from build123d import *

# Parameters (mm, degrees)
SKETCH1_R             = 1.55
BOSS_EXTRUDE1_DEPTH   = 1.6
SKETCH1_3_R           = 1.55
BOSS_EXTRUDE2_DEPTH   = 4
BOSS_EXTRUDE2_2_DEPTH = 4
BOSS_EXTRUDE2_3_DEPTH = 4
BOSS_EXTRUDE2_4_DEPTH = 4
SKETCH1_4_R           = 1.55
BOSS_EXTRUDE3_DEPTH   = 17.6
BOSS_EXTRUDE4_START   = 12
SKETCH2_W             = 26.677983171
SKETCH2_H             = 36.175587157
BOSS_EXTRUDE4_DEPTH   = 1.6


with BuildPart() as part:
    # Sketch1 → Boss-Extrude1 (new body)
    with BuildSketch(Plane.XY):
        Polygon((72, 55), (70, 55), (70, 65), (0, 65), (0, 0), (70, 0), (70, 35), (72, 35), align=None)
        with Locations((3.5, 3.5)):
            Circle(SKETCH1_R, mode=Mode.SUBTRACT)
        with Locations((66.5, 3.5)):
            Circle(SKETCH1_R, mode=Mode.SUBTRACT)
        with Locations((45.06, 30.1)):
            Circle(SKETCH1_R, mode=Mode.SUBTRACT)
        with Locations((65.76, 30.1)):
            Circle(SKETCH1_R, mode=Mode.SUBTRACT)
        with Locations((3.523, 61.1)):
            Circle(SKETCH1_R, mode=Mode.SUBTRACT)
        with Locations((45.06, 61.1)):
            Circle(SKETCH1_R, mode=Mode.SUBTRACT)
        with Locations((65.76, 61.1)):
            Circle(SKETCH1_R, mode=Mode.SUBTRACT)
    extrude(amount=BOSS_EXTRUDE1_DEPTH)



with BuildPart() as body_2:
    # Sketch1_3 → Boss-Extrude2 (new body)
    with BuildSketch(Plane.XY):
        with Locations((65.76, 30.1)):
            Circle(SKETCH1_3_R)
    extrude(amount=-BOSS_EXTRUDE2_DEPTH)


with BuildPart() as body_3:
    # Sketch1_3 → Boss-Extrude2 2 (new body)
    with BuildSketch(Plane.XY):
        with Locations((45.06, 61.1)):
            Circle(SKETCH1_3_R)
    extrude(amount=-BOSS_EXTRUDE2_2_DEPTH)


with BuildPart() as body_4:
    # Sketch1_3 → Boss-Extrude2 3 (new body)
    with BuildSketch(Plane.XY):
        with Locations((65.76, 61.1)):
            Circle(SKETCH1_3_R)
    extrude(amount=-BOSS_EXTRUDE2_3_DEPTH)


with BuildPart() as body_5:
    # Sketch1_3 → Boss-Extrude2 4 (new body)
    with BuildSketch(Plane.XY):
        with Locations((45.06, 30.1)):
            Circle(SKETCH1_3_R)
    extrude(amount=-BOSS_EXTRUDE2_4_DEPTH)


with BuildPart() as part_1:
    add(part.part)

    add(body_2.part)  # Boss-Extrude3 merges body 2

    add(body_3.part)  # Boss-Extrude3 merges body 3

    add(body_4.part)  # Boss-Extrude3 merges body 4

    add(body_5.part)  # Boss-Extrude3 merges body 5
    # Sketch1_4 → Boss-Extrude3 (add)
    with BuildSketch(Plane.XY):
        with Locations((45.06, 61.1)):
            Circle(SKETCH1_4_R)
        with Locations((65.76, 61.1)):
            Circle(SKETCH1_4_R)
        with Locations((45.06, 30.1)):
            Circle(SKETCH1_4_R)
        with Locations((65.76, 30.1)):
            Circle(SKETCH1_4_R)
    extrude(amount=BOSS_EXTRUDE3_DEPTH)

    # Sketch2 → Boss-Extrude4 (add)
    with BuildSketch(Plane.XY.offset(1.6).offset(BOSS_EXTRUDE4_START)):
        with Locations((55.356329563, 45.415531536)):
            Rectangle(SKETCH2_W, SKETCH2_H)
    extrude(amount=BOSS_EXTRUDE4_DEPTH)


solid = part_1.part
Work out the finished part from the listing and answer in its coordinate system (mm). A direction names the side the tool comes from. Round coordinates to 2 decimals unless told otherwise and drop trailing zeros. Write each loop counter-clockwise with the first axis right and the second up, starting at its lowest first coordinate (ties: lowest second). Pieces come first, ordered by that corner, then holes. Notation, with made-up numbers: (27, -22) - (55, -22) arc R24 ccw to (55, 5) - close; hole circle Ø8 at (-29.75, -13). An arc over 180 degrees is marked (long way). Answer in a Markdown table with one row per item. Add a question column.
1. A cutting plane is placed at A-A, the plane y = 36.5. Determine the outline of the cut face in (x, z).
2. The mould has two halves that part along X. Classify faces 5 (the cylindrical face through (67.238, 30.566, 16.383)), 6 (the flat face through (70, 60, 1)), 7 (the flat face through (45, 61, 17.6)): +X half, -X half, draft (parallel to the pull), parting line (faces both ways), or undercut.
3. A cutting plane is placed at B-B, the plane x = 50. Determine the outline of the cut face in (y, z).
4. For faces 1 (the flat face through (70, 17, 1)), 2 (the cylindrical face through (46.538, 30.566, 7.516)), 3 (the cylindrical face through (46.538, 30.566, 16.383)), 4 (the cylindrical face through (46.538, 30.566, -1.972)), determine the directions among +Z, -Z, +X, -X, +Y, -Y from which every point of the face is accessible in a straight line to the end or side of a thin tool.
5. Find the intervals of material crossed by line 1 along Y through (x, z) = (66.5, 1.2); line 2 along Z through (x, y) = (51, 52); line 3 along Y through (x, z) = (3.5, 0.6), in increasing order. Write a range as from..to.
6. Given pin 1 (8 mm diameter, centred on x = 20.5, y = 56.5, fed in from -Z); pin 2 (1.3 mm diameter, centred on x = 53.5, z = 14.5, fed in from +Y); pin 3 (1.8 mm diameter, centred on y = 62.5, z = 1, fed in from +X), each flat-ended and moving along its own axis, determine where each tip first touches the part or whether it passes through.
7. A cutting plane is placed at D-D, the plane z = 4.5. Determine the outline of the cut face in (x, y), and give its area (3 significant figures).
8. A cutting plane is placed at C-C, the plane y = 3.5. Determine the outline of the cut face in (x, z), and give its area (3 significant figures).
Worked out:
| question | item | result |
|---|---|---|
| 1 | outline | (0, 0) - (72, 0) - (72, 1.6) - (0, 1.6) - close; (42.02, 13.6) - (68.7, 13.6) - (68.7, 15.2) - (42.02, 15.2) - close |
| 2 | face 5 | undercut |
| 2 | face 6 | +X half |
| 2 | face 7 | draft |
| 3 | outline | (0, 0) - (65, 0) - (65, 1.6) - (0, 1.6) - close; (27.33, 13.6) - (63.5, 13.6) - (63.5, 15.2) - (27.33, 15.2) - close |
| 4 | face 1 | +Z, -Z, +X, -Y |
| 4 | face 2 | none |
| 4 | face 3 | +Z |
| 4 | face 4 | -Z |
| 5 | line 1 | 0..1.95, 5.05..65 |
| 5 | line 2 | 0..1.6, 13.6..15.2 |
| 5 | line 3 | 0..1.95, 5.05..59.55, 62.65..65 |
| 6 | pin 1 | z = 0 |
| 6 | pin 2 | y = 63.5 |
| 6 | pin 3 | x = 70 |
| 7 | outline | circle Ø3.1 at (45.06, 30.1); circle Ø3.1 at (45.06, 61.1); circle Ø3.1 at (65.76, 30.1); circle Ø3.1 at (65.76, 61.1) |
| 7 | area | 30.2 mm^2 |
| 8 | outline | (0, 0) - (1.95, 0) - (1.95, 1.6) - (0, 1.6) - close; (5.05, 0) - (64.95, 0) - (64.95, 1.6) - (5.05, 1.6) - close; (68.05, 0) - (70, 0) - (70, 1.6) - (68.05, 1.6) - close |
| 8 | area | 102 mm^2 |
